Job drawing, mm, ordinate dimensions from the low corner. One solid piece. A direction names the side the tool comes from. Give positions to 0.01 mm unless a question says otherwise; leave off trailing zeros. Order: outer loops, then holes, each group sorted by start corner. A loop starts at its lowest first (then second) coordinate and runs counter-clockwise, first axis right, second up. Notation, with made-up numbers: (-10, 18.25) - (28, 18.25) arc R27 ccw to (28, 53.25) - close; hole circle Ø10 at (60, 7). An arc over 180 degrees is marked (long way). Write each question's results on one line, items separated by ' | '. Start each with the question number.
1) Cut at A-A on z = 4.5. List the corners of the cut face in (x, y), plus the area to 3 significant figures.
2) Tool access for the marked faces 1, 2 and 3: list every direction of +Z, -Z, +X, -X, +Y, -Y with a clear straight run to the whole face (end or side of a thin tool).
3) Cut at C-C on x = 3.2. List the corners of the cut face in (y, z).
4) Drop flat-ended pins along their axis: pin 1 Ø5 at (y, z) = (4, 4.5) entering from +X; pin 2 Ø1.5 at (x, z) = (2.5, 7.5) entering from -Y; pin 3 Ø2.5 at (y, z) = (4.5, 4.5) entering from -X; pin 4 Ø2 at (x, z) = (3, 6) entering from +Y. Give the stop position or say it passes through.
5) Drill centre lines: line 1 along Z through (x, y) = (3.4, 4.5); line 2 along X through (y, z) = (2.25, 3.25); line 3 along Y through (x, z) = (5.2, 5). Where is each one in solid material? Low to high. Write a range as from..to.
6) Two-plate mould, pull along Y, no slides. Class the marked faces 4, 5 and 6: +Y half, -Y half, draft (parallel to the pull), parting line (faces both ways), or undercut.
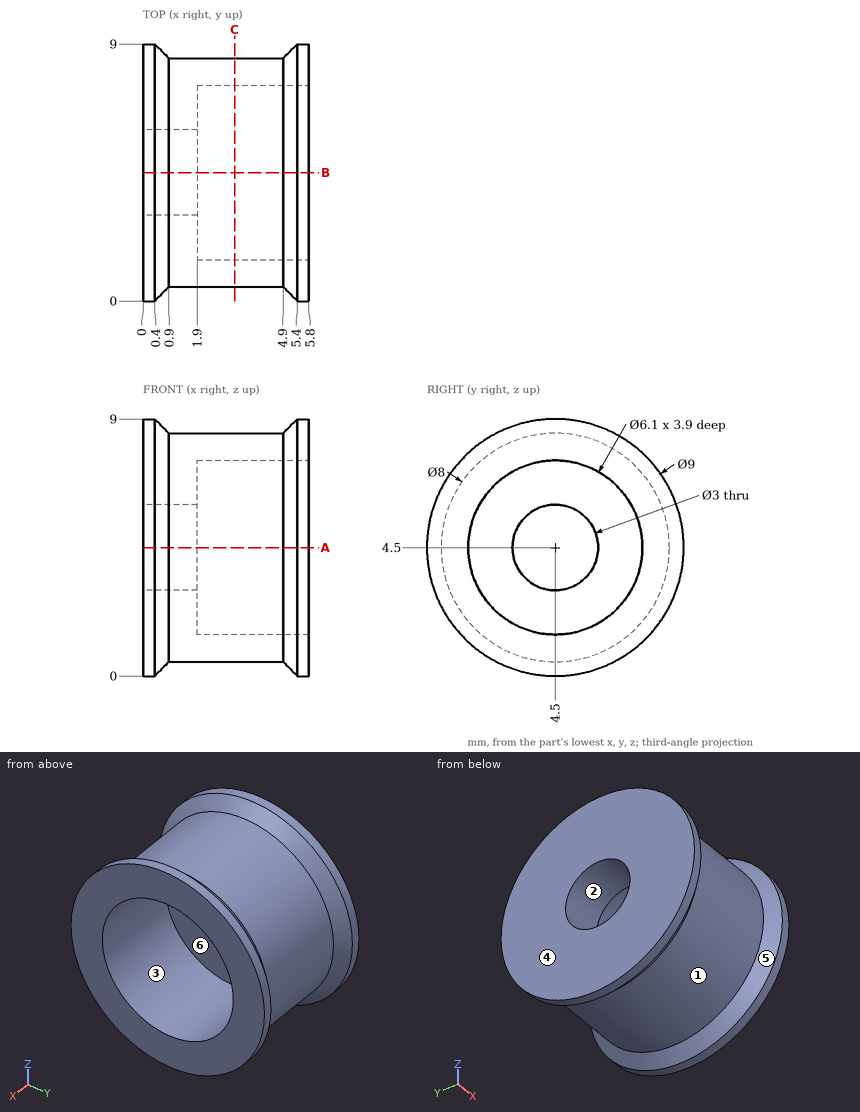
Results:
1) outline: (0, 0) - (0.4, 0) - (0.9, 0.5) - (4.9, 0.5) - (5.4, 0) - (5.8, 0) - (5.8, 1.45) - (1.9, 1.45) - (1.9, 3) - (0, 3) - close; (0, 6) - (1.9, 6) - (1.9, 7.55) - (5.8, 7.55) - (5.8, 9) - (5.4, 9) - (4.9, 8.5) - (0.9, 8.5) - (0.4, 9) - (0, 9) - close | area: 18.2 mm^2
2) face 1: none | face 2: +X, -X | face 3: +X
3) outline: circle Ø8 at (4.5, 4.5); hole circle Ø6.1 at (4.5, 4.5)
4) pin 1: x = 1.9 | pin 2: y = 1.19 | pin 3: through | pin 4: y = 8.47
5) line 1: 0.5..1.45, 7.55..8.5 | line 2: 0..1.9 | line 3: 0.23..1.49, 7.51..8.77
6) face 4: draft | face 5: parting line | face 6: undercut
